from build123d import *

# Parameters (mm, degrees)
SKETCH1_R            = 5
BOSS_EXTRUDE1_DEPTH  = 6.1
M3_CLEARANCE_HOLE1_D = 3.2
SKETCH4_R            = 5.808101239
SKETCH4_R_2          = 2.5
CUT_EXTRUDE1_DEPTH   = 5.1


with BuildPart() as part:
    # Sketch1 → Boss-Extrude1 (new body)
    with BuildSketch(Plane(origin=(0, 0, 0), x_dir=(1, 0, 0), z_dir=(0, 1, 0))):
        with Locations(Location((0, 0, 0), (0, 0, 270))):
            Circle(SKETCH1_R)
    extrude(amount=BOSS_EXTRUDE1_DEPTH)

    # M3 Clearance Hole1 (through all)
    with Locations(Plane(origin=(0, 6.1, 0), x_dir=(-1, 0, 0), z_dir=(0, 1, 0))):
        with Locations((0, 0)):
            Hole(M3_CLEARANCE_HOLE1_D / 2)

    # Sketch4 → Cut-Extrude1 (cut)
    with BuildSketch(Plane(origin=(0, 6.1, 0), x_dir=(1, 0, 0), z_dir=(0, 1, 0))):
        Circle(SKETCH4_R)
        with Locations(Location((0, 0, 0), (0, 0, 270))):
            Circle(SKETCH4_R_2, mode=Mode.SUBTRACT)
    extrude(amount=-CUT_EXTRUDE1_DEPTH, mode=Mode.SUBTRACT)


solid = part.part
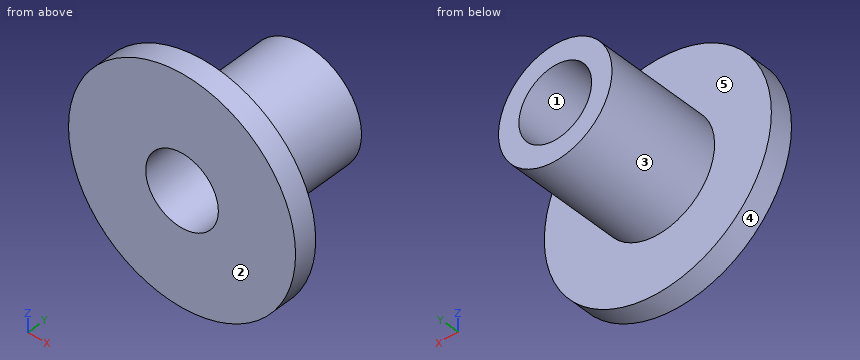
Verification items for the finished model (mm, model axes). Face numbers are marked on the shaded views. A direction names the side the tool comes from. Give positions to 0.01 mm unless a question says otherwise; leave off trailing zeros. Write each loop counter-clockwise with the first axis right and the second up, starting at its lowest first coordinate (ties: lowest second). Pieces come first, ordered by that corner, then holes. Notation, with made-up numbers: M -3.5,71.25 L 6.5,71.25 A24 ccw 6.5,92.25 Z; hole C 50.5,52 d1. An arc over 180 degrees is marked long. Write item = value, one per line.
(1) Material ranges on line 1 (Z direction, x = 0, y = 0.5); line 2 (Y direction, x = 3, z = -3.75); line 3 (Z direction, x = -1, y = 5), recorded low to high.
Found:
line_1 = -5 to -1.6, 1.6 to 5
line_2 = 0 to 1
line_3 = -2.29 to -1.25, 1.25 to 2.29
(2) Sectioned sample at B-B (y = 0.75). Record the cut outline in (x, z), then the cut area to 3 significant figures.
Found:
outline = C 0,0 d10; hole C 0,0 d3.2
area = 70.5 mm2
(3) Sectioned sample at D-D (z = 4). Record the cut outline in (x, y).
Found:
outline = M -3,0 L 3,0 L 3,1 L -3,1 Z
(4) Draft check along Z on the marked faces 1, 2 and 3. Enter one of: released by +Z, released by -Z, zero draft, split by the parting line, or undercut.
Found:
face_1 = undercut
face_2 = zero draft
face_3 = split by the parting line
(5) Sectioned sample at A-A (z = 0). Record the cut outline in (x, y), then the cut area to 3 significant figures.
Found:
outline = M -5,0 L -1.6,0 L -1.6,6.1 L -2.5,6.1 L -2.5,1 L -5,1 Z; M 1.6,0 L 5,0 L 5,1 L 2.5,1 L 2.5,6.1 L 1.6,6.1 Z
area = 16.0 mm2
(6) Go/stop test with flat-tipped pins: pin 1 Ø2 at (y, z) = (2.5, -1.5) entering from +X; pin 2 Ø6 at (x, z) = (-2, -0.5) entering from -Y; pin 3 Ø1 at (y, z) = (4.5, 2) entering from -X; pin 4 Ø1.5 at (y, z) = (0.5, 2) entering from -X. Record where each tip stops, or that it passes through.
Found:
pin_1 = 2.45
pin_2 = 0
pin_3 = -2
pin_4 = -4.84
(7) Sectioned sample at C-C (x = -2). Record the cut outline in (y, z).
Found:
outline = M 0,-4.58 L 1,-4.58 L 1,-1.5 L 6.1,-1.5 L 6.1,1.5 L 1,1.5 L 1,4.58 L 0,4.58 Z
(8) Access from +Z, -Z, +X, -X, +Y, -Y to the whole of each face (thin tool, end or side, straight path). Record for the marked faces 4 and 5.
Found:
face_4 = +Y, -Y
face_5 = +Y
